Read the model definition and answer for the solid it produces. Units are mm, in the model's axes. A direction names the side the tool comes from. Coordinates: 2 decimals unless noted, no trailing zeros.
1) Each of these flat-tipped pins is pushed along its axis until it touches: pin 1 Ø3 at (x, y) = (-0.5, 1) entering from +Z; pin 2 Ø3 at (x, y) = (-0.5, 1) entering from -Z; pin 3 Ø1.5 at (y, z) = (-1.5, 3.5) entering from -X. Where does it stop, or does it pass through?
2) Which of the six approach directions +Z, -Z, +X, -X, +Y, -Y give full straight-line access (tool end or side, diameter ignored) to faces 1 (the face through (-3.65, -5.04, 12.32)), 2 (the face through (-3.633, 5.028, 12.325)), 3 (the face through (4.8, -3.96, 12.32)), 4 (the face through (-6.192, -0.373, 12.325)), 5 (the face through (-5.623, -2.658, 12.325))?
3) Find the intervals of material crossed by line 1 (Y direction, x = 0, z = -0.55); line 2 (Y direction, x = 0, z = -3.85); line 3 (X direction, y = 6, z = 22.5), in increasing order.
from build123d import *

# Parameters (mm, degrees)
EXTRUDE_1_DEPTH     = 25
SKETCH_2_R          = 5
SKETCH_2_R_2        = 2.75
EXTRUDE_2_DEPTH     = 5
SKETCH_3_R          = 3
EXTRUDE_3_DEPTH     = 1.5
SKETCH_4_R          = 3
CUT_EXTRUDE_1_DEPTH = 23.5
SKETCH_5_R          = 1.6
CUT_EXTRUDE_2_DEPTH = 26.363528361


with BuildPart() as part:
    # 草图1 → 凸台-拉伸1 (new body)
    with BuildSketch(Plane.XY):
        with BuildLine():
            ThreePointArc((-0.126349393, 5.623580784), (-0.353196672, 5.613900347), (-0.579468474, 5.595072947))
            ThreePointArc((-0.579468474, 5.595072947), (-0.765010507, 6.164212032), (-1.101088476, 6.659587387))
            ThreePointArc((-1.101088476, 6.659587387), (-1.264823873, 6.630438942), (-1.427791454, 6.597265461))
            ThreePointArc((-1.427791454, 6.597265461), (-1.557909016, 6.012958552), (-1.520907565, 5.415483836))
            ThreePointArc((-1.520907565, 5.415483836), (-1.738220593, 5.349692904), (-1.952701466, 5.275185493))
            ThreePointArc((-1.952701466, 5.275185493), (-2.27395349, 5.7803016), (-2.722667793, 6.176534634))
            ThreePointArc((-2.722667793, 6.176534634), (-2.874010218, 6.107582604), (-3.023607963, 6.03492294))
            ThreePointArc((-3.023607963, 6.03492294), (-3.004326424, 5.436614185), (-2.819901521, 4.867112122))
            ThreePointArc((-2.819901521, 4.867112122), (-3.014025722, 4.749344581), (-3.203239044, 4.623838733))
            ThreePointArc((-3.203239044, 4.623838733), (-3.640015612, 5.033193559), (-4.173171879, 5.305387495))
            ThreePointArc((-4.173171879, 5.305387495), (-4.302611931, 5.200964389), (-4.429440063, 5.093384015))
            ThreePointArc((-4.429440063, 5.093384015), (-4.261970953, 4.518667354), (-3.941710694, 4.012921854))
            ThreePointArc((-3.941710694, 4.012921854), (-4.100448529, 3.850577471), (-4.252505332, 3.68195918))
            ThreePointArc((-4.252505332, 3.68195918), (-4.777362166, 3.969831456), (-5.361460228, 4.100883347))
            ThreePointArc((-5.361460228, 4.100883347), (-5.460864712, 3.967550453), (-5.556954155, 3.831809041))
            ThreePointArc((-5.556954155, 3.831809041), (-5.251820172, 3.316796034), (-4.815847687, 2.906584947))
            ThreePointArc((-4.815847687, 2.906584947), (-4.929225075, 2.709864417), (-5.03457107, 2.508728591))
            ThreePointArc((-5.03457107, 2.508728591), (-5.614529486, 2.657030243), (-6.212868313, 2.638705616))
            ThreePointArc((-6.212868313, 2.638705616), (-6.27599128, 2.484840731), (-6.335304379, 2.329467412))
            ThreePointArc((-6.335304379, 2.329467412), (-5.911678216, 1.906518221), (-5.387387259, 1.617616618))
            ThreePointArc((-5.387387259, 1.617616618), (-5.448280281, 1.398880615), (-5.500296192, 1.177865357))
            ThreePointArc((-5.500296192, 1.177865357), (-6.098915269, 1.177278047), (-6.673899032, 1.010728308))
            ThreePointArc((-6.673899032, 1.010728308), (-6.696774234, 0.845999327), (-6.71558413, 0.680756778))
            ThreePointArc((-6.71558413, 0.680756778), (-6.200083775, 0.376446857), (-5.620417476, 0.227007488))
            ThreePointArc((-5.620417476, 0.227007488), (-5.625, 0), (-5.620417476, -0.227007488))
            ThreePointArc((-5.620417476, -0.227007488), (-6.200083775, -0.376446857), (-6.71558413, -0.680756778))
            ThreePointArc((-6.71558413, -0.680756778), (-6.696774234, -0.845999327), (-6.673899032, -1.010728308))
            ThreePointArc((-6.673899032, -1.010728308), (-6.098915269, -1.177278047), (-5.500296192, -1.177865357))
            ThreePointArc((-5.500296192, -1.177865357), (-5.448280281, -1.398880615), (-5.387387259, -1.617616618))
            ThreePointArc((-5.387387259, -1.617616618), (-5.911678216, -1.906518221), (-6.335304379, -2.329467412))
            ThreePointArc((-6.335304379, -2.329467412), (-6.27599128, -2.484840731), (-6.212868313, -2.638705616))
            ThreePointArc((-6.212868313, -2.638705616), (-5.614529486, -2.657030243), (-5.03457107, -2.508728591))
            ThreePointArc((-5.03457107, -2.508728591), (-4.929225075, -2.709864417), (-4.815847687, -2.906584947))
            ThreePointArc((-4.815847687, -2.906584947), (-5.251820172, -3.316796034), (-5.556954155, -3.831809041))
            ThreePointArc((-5.556954155, -3.831809041), (-5.460864712, -3.967550453), (-5.361460228, -4.100883347))
            ThreePointArc((-5.361460228, -4.100883347), (-4.777362166, -3.969831456), (-4.252505332, -3.68195918))
            ThreePointArc((-4.252505332, -3.68195918), (-4.100448529, -3.850577471), (-3.941710694, -4.012921854))
            ThreePointArc((-3.941710694, -4.012921854), (-4.261970953, -4.518667354), (-4.429440063, -5.093384015))
            ThreePointArc((-4.429440063, -5.093384015), (-4.302611931, -5.200964389), (-4.173171879, -5.305387495))
            ThreePointArc((-4.173171879, -5.305387495), (-3.640015612, -5.033193559), (-3.203239044, -4.623838733))
            ThreePointArc((-3.203239044, -4.623838733), (-3.014025722, -4.749344581), (-2.819901521, -4.867112122))
            ThreePointArc((-2.819901521, -4.867112122), (-3.004326424, -5.436614185), (-3.023607963, -6.03492294))
            ThreePointArc((-3.023607963, -6.03492294), (-2.874010218, -6.107582604), (-2.722667793, -6.176534634))
            ThreePointArc((-2.722667793, -6.176534634), (-2.27395349, -5.7803016), (-1.952701466, -5.275185493))
            ThreePointArc((-1.952701466, -5.275185493), (-1.738220593, -5.349692904), (-1.520907565, -5.415483836))
            ThreePointArc((-1.520907565, -5.415483836), (-1.557909016, -6.012958552), (-1.427791454, -6.597265461))
            ThreePointArc((-1.427791454, -6.597265461), (-1.264823873, -6.630438942), (-1.101088476, -6.659587387))
            ThreePointArc((-1.101088476, -6.659587387), (-0.765010507, -6.164212032), (-0.579468474, -5.595072947))
            ThreePointArc((-0.579468474, -5.595072947), (-0.353196672, -5.613900347), (-0.126349393, -5.623580784))
            ThreePointArc((-0.126349393, -5.623580784), (-0.013602456, -6.21148662), (0.257738444, -6.745077531))
            ThreePointArc((0.257738444, -6.745077531), (0.423836007, -6.736680417), (0.589676279, -6.724193772))
            ThreePointArc((0.589676279, -6.724193772), (0.7920009, -6.160802353), (0.830174654, -5.563401392))
            ThreePointArc((0.830174654, -5.563401392), (1.054019895, -5.525365785), (1.276147777, -5.478327469))
            ThreePointArc((1.276147777, -5.478327469), (1.531558797, -6.019724139), (1.927073686, -6.469071572))
            ThreePointArc((1.927073686, -6.469071572), (2.085864712, -6.419631485), (2.243389504, -6.366294333))
            ThreePointArc((2.243389504, -6.366294333), (2.299247977, -5.770286804), (2.187654855, -5.182160866))
            ThreePointArc((2.187654855, -5.182160866), (2.395008515, -5.08965217), (2.598459887, -4.988850691))
            ThreePointArc((2.598459887, -4.988850691), (2.980486578, -5.449720251), (3.475323802, -5.786590055))
            ThreePointArc((3.475323802, -5.786590055), (3.616830866, -5.699213497), (3.756142317, -5.608377207))
            ThreePointArc((3.756142317, -5.608377207), (3.662024848, -5.017202913), (3.407676656, -4.475306114))
            ThreePointArc((3.407676656, -4.475306114), (3.585509942, -4.334136991), (3.757501207, -4.185906076))
            ThreePointArc((3.757501207, -4.185906076), (4.242139425, -4.537290397), (4.805206542, -4.740515804))
            ThreePointArc((4.805206542, -4.740515804), (4.920538235, -4.620692965), (5.032882894, -4.498065115))
            ThreePointArc((5.032882894, -4.498065115), (4.79470323, -3.948869711), (4.4135816, -3.48725142))
            ThreePointArc((4.4135816, -3.48725142), (4.550720593, -3.306292044), (4.680444907, -3.119945588))
            ThreePointArc((4.680444907, -3.119945588), (5.237243052, -3.339765901), (5.833160483, -3.39657751))
            ThreePointArc((5.833160483, -3.39657751), (5.91507009, -3.2518373), (5.993388929, -3.105123049))
            ThreePointArc((5.993388929, -3.105123049), (5.626112774, -2.632414502), (5.14216498, -2.280079894))
            ThreePointArc((5.14216498, -2.280079894), (5.229992733, -2.070700609), (5.30929904, -1.857947445))
            ThreePointArc((5.30929904, -1.857947445), (5.903271436, -1.93239163), (6.494595498, -1.839219759))
            ThreePointArc((6.494595498, -1.839219759), (6.537936338, -1.678656738), (6.577308295, -1.517074682))
            ThreePointArc((6.577308295, -1.517074682), (6.104012961, -1.150555009), (5.547647223, -0.929642562))
            ThreePointArc((5.547647223, -0.929642562), (5.580645195, -0.704999439), (5.604550388, -0.47920763))
            ThreePointArc((5.604550388, -0.47920763), (6.198375565, -0.403598087), (6.747951192, -0.166297067))
            ThreePointArc((6.747951192, -0.166297067), (6.75, 0), (6.747951192, 0.166297067))
            ThreePointArc((6.747951192, 0.166297067), (6.198375565, 0.403598087), (5.604550388, 0.47920763))
            ThreePointArc((5.604550388, 0.47920763), (5.580645195, 0.704999439), (5.547647223, 0.929642562))
            ThreePointArc((5.547647223, 0.929642562), (6.104012961, 1.150555009), (6.577308295, 1.517074682))
            ThreePointArc((6.577308295, 1.517074682), (6.537936338, 1.678656738), (6.494595498, 1.839219759))
            ThreePointArc((6.494595498, 1.839219759), (5.903271436, 1.93239163), (5.30929904, 1.857947445))
            ThreePointArc((5.30929904, 1.857947445), (5.229992733, 2.070700609), (5.14216498, 2.280079894))
            ThreePointArc((5.14216498, 2.280079894), (5.626112774, 2.632414502), (5.993388929, 3.105123049))
            ThreePointArc((5.993388929, 3.105123049), (5.91507009, 3.2518373), (5.833160483, 3.39657751))
            ThreePointArc((5.833160483, 3.39657751), (5.237243052, 3.339765901), (4.680444907, 3.119945588))
            ThreePointArc((4.680444907, 3.119945588), (4.550720593, 3.306292044), (4.4135816, 3.48725142))
            ThreePointArc((4.4135816, 3.48725142), (4.79470323, 3.948869711), (5.032882894, 4.498065115))
            ThreePointArc((5.032882894, 4.498065115), (4.920538235, 4.620692965), (4.805206542, 4.740515804))
            ThreePointArc((4.805206542, 4.740515804), (4.242139425, 4.537290397), (3.757501207, 4.185906076))
            ThreePointArc((3.757501207, 4.185906076), (3.585509942, 4.334136991), (3.407676656, 4.475306114))
            ThreePointArc((3.407676656, 4.475306114), (3.662024848, 5.017202913), (3.756142317, 5.608377207))
            ThreePointArc((3.756142317, 5.608377207), (3.616830866, 5.699213497), (3.475323802, 5.786590055))
            ThreePointArc((3.475323802, 5.786590055), (2.980486578, 5.449720251), (2.598459887, 4.988850691))
            ThreePointArc((2.598459887, 4.988850691), (2.395008515, 5.08965217), (2.187654855, 5.182160866))
            ThreePointArc((2.187654855, 5.182160866), (2.299247977, 5.770286804), (2.243389504, 6.366294333))
            ThreePointArc((2.243389504, 6.366294333), (2.085864712, 6.419631485), (1.927073686, 6.469071572))
            ThreePointArc((1.927073686, 6.469071572), (1.531558797, 6.019724139), (1.276147777, 5.478327469))
            ThreePointArc((1.276147777, 5.478327469), (1.054019895, 5.525365785), (0.830174654, 5.563401392))
            ThreePointArc((0.830174654, 5.563401392), (0.7920009, 6.160802353), (0.589676279, 6.724193772))
            ThreePointArc((0.589676279, 6.724193772), (0.423836007, 6.736680417), (0.257738444, 6.745077531))
            ThreePointArc((0.257738444, 6.745077531), (-0.013602456, 6.21148662), (-0.126349393, 5.623580784))
        make_face()
    extrude(amount=EXTRUDE_1_DEPTH)

    # 草图2 → 凸台-拉伸2 (add)
    with BuildSketch(Plane(origin=(0, 0, 0), x_dir=(-1, 0, 0), z_dir=(0, 0, -1))):
        with Locations(Location((0, 0, 0), (0, 0, 180))):
            Circle(SKETCH_2_R)
        Circle(SKETCH_2_R_2, mode=Mode.SUBTRACT)
    extrude(amount=EXTRUDE_2_DEPTH)

    # 草图3 → 凸台-拉伸3 (add)
    with BuildSketch(Plane(origin=(0, 0, 0), x_dir=(-1, 0, 0), z_dir=(0, 0, -1))):
        Circle(SKETCH_3_R)
    extrude(amount=EXTRUDE_3_DEPTH)

    # 草图4 → 切除-拉伸1 (cut)
    with BuildSketch(Plane.XY.offset(25)):
        Circle(SKETCH_4_R)
    extrude(amount=-CUT_EXTRUDE_1_DEPTH, mode=Mode.SUBTRACT)

    # 草图5 → 切除-拉伸2 (cut, through all)
    with BuildSketch(Plane.XY.offset(1.5)):
        Circle(SKETCH_5_R)
    extrude(amount=-CUT_EXTRUDE_2_DEPTH, mode=Mode.SUBTRACT)


solid = part.part
Reported:
1. pin 1: stops at z = 1.5
1. pin 2: stops at z = -1.5
1. pin 3: stops at x = -6.71
2. face 1: +Z, -Z, -Y
2. face 2: +Z, -Z, +Y
2. face 3: +Z, -Z, +X
2. face 4: +Z, -Z, -X
2. face 5: +Z, -Z
3. line 1: y = -5 to -1.6, 1.6 to 5
3. line 2: y = -5 to -2.75, 2.75 to 5
3. line 3: x = -3.03 to -2.49, -1.56 to -0.69, -0.07 to 0.82, 1.52 to 2.3
